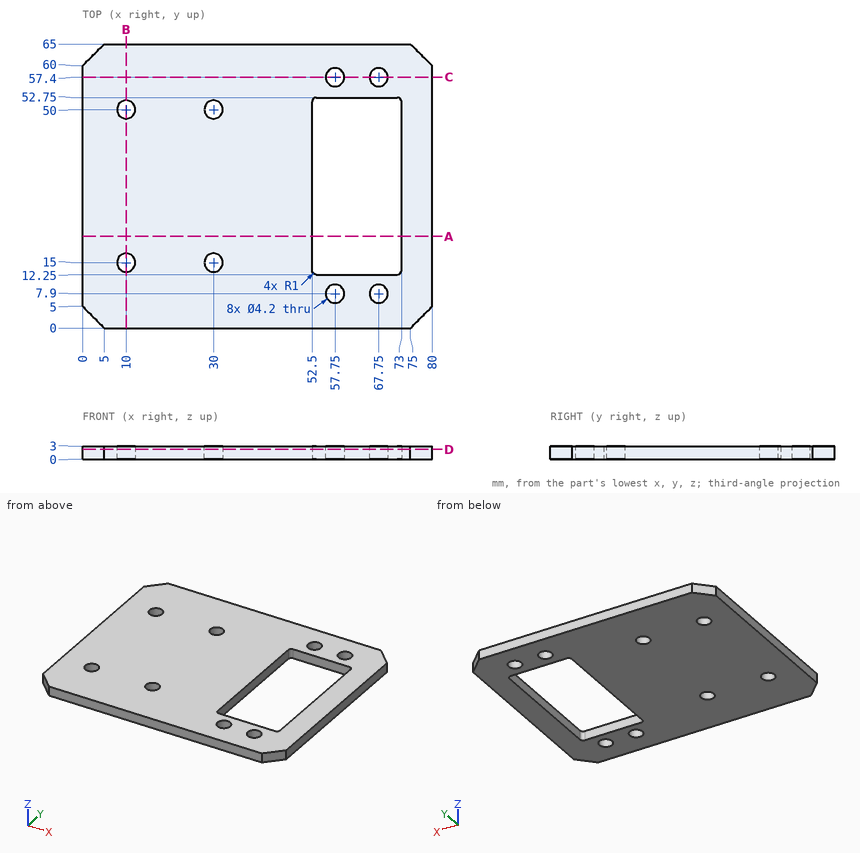
Print and shaded views of the part. All mm, measured from the part's lowest x, y and z. Round coordinates to 2 decimals unless told otherwise and drop trailing zeros. Write each loop counter-clockwise with the first axis right and the second up, starting at its lowest first coordinate (ties: lowest second). Pieces come first, ordered by that corner, then holes. Notation, with made-up numbers: M 3.25,-16 L 28.25,-16 A13 cw 28.25,-4 Z; hole C -2.5,73.5 d1. An arc over 180 degrees is marked long. One line per question, with ' | ' between items.
(1) Saw through at B-B on x = 10. Write the cut outline in (y, z).
Answer key:
outline: M 0,0 L 12.9,0 L 12.9,3 L 0,3 Z; M 17.1,0 L 47.9,0 L 47.9,3 L 17.1,3 Z; M 52.1,0 L 65,0 L 65,3 L 52.1,3 Z
(2) Saw through at C-C on y = 57.4. Write the cut outline in (x, z), then the cut area to 3 significant figures.
Answer key:
outline: M 0,0 L 55.65,0 L 55.65,3 L 0,3 Z; M 59.85,0 L 65.65,0 L 65.65,3 L 59.85,3 Z; M 69.85,0 L 80,0 L 80,3 L 69.85,3 Z | area: 215 mm^2
(3) Probe line 1 along Y through (x, z) = (30, 0.25); line 2 along Y through (x, z) = (57.75, 1.4); line 3 along X through (y, z) = (27, 1.35). List the from-to ranges inside material, lowest first.
Answer key:
line 1: y = 0 to 12.9, 17.1 to 47.9, 52.1 to 65 | line 2: y = 0 to 5.8, 10 to 12.25, 52.75 to 55.3, 59.5 to 65 | line 3: x = 0 to 52.5, 73 to 80
(4) Saw through at A-A on y = 21. Write the cut outline in (x, z), then the cut area to 4 significant figures.
Answer key:
outline: M 0,0 L 52.5,0 L 52.5,3 L 0,3 Z; M 73,0 L 80,0 L 80,3 L 73,3 Z | area: 178.5 mm^2
(5) Saw through at D-D on z = 2.3. Count the separate pieces of the cut face and the enclosed holes in it, then the cut area to 3 significant figures.
Answer key:
separate pieces: 1 | enclosed holes: 9 | area: 4,210 mm^2
